Autodesk Inventor part; units mm, degrees
ref_plane "YZ Plane" through (0, 0, 0) normal (1, 0, 0) x (0, 1, 0)
ref_plane "XZ Plane" through (0, 0, 0) normal (0, 1, 0) x (-1, 0, 0)
ref_plane "XY Plane" through (0, 0, 0) normal (0, 0, 1) x (1, 0, 0)
sketch "Sketch1" plane through (0, 0, 0) normal (0, 1, 0) x (-1, 0, 0)
  line L0 (0, 0) -> (50.8, 0)
  line L1 (50.8, 0) -> (50.8, -50.8)
  line L2 (50.8, -50.8) -> (0, -50.8)
  line L3 (0, -50.8) -> (0, 0)
  dimension "d0" = 50.8
  dimension "d1" = 50.8
extrude "Extrusion1" add sketch "Sketch1" along normal blind 3.175
sketch "Sketch2" plane through (0, 3.175, 0) normal (0, 1, 0) x (1, 0, 0)
  line L0 (-50.8, 0) -> (0, 0)
  line L1 (0, 0) -> (0, 50.8)
  line L2 (-50.8, 0) -> (0, 0)
  line L3 (0, 0) -> (0, 3.175)
  line L4 (0, 3.175) -> (-50.8, 3.175)
  line L5 (-50.8, 3.175) -> (-50.8, 0)
  dimension "d4" = 3.175
extrude "Extrusion2" add sketch "Sketch2" along normal blind 22.225
sketch "Sketch3" plane through (0, 3.175, 0) normal (0, 1, 0) x (1, 0, 0)
  line L0 (0, 3.175) -> (0, 50.8)
  line L1 (-50.8, 50.8) -> (-50.8, 3.175)
  line L2 (0, 50.8) -> (-50.8, 50.8)
  point P0 (0, 0)
  point P1 (-12.7, 41.656)
  point P2 (-38.1, 41.656)
  dimension "d9" = 9.144
  dimension "d10" = 9.144
  dimension "d18" = 25.4
  dimension "d19" = 12.7
  dimension "d20" = 12.7
  dimension "d21" = 50.8
hole "Hole1" at (-12.7, 3.175, -41.656) at (-38.1, 3.175, -41.656) direction (0, -1, 0) diameter 6.35 depth 25.4 tip angle 118
sketch "Sketch5" plane through (-50.8, 0, 0) normal (0, 0, 1) x (1, 0, 0)
  line L0 (0, 25.4) -> (50.8, 25.4)
  line L1 (50.8, 0) -> (50.8, 25.4)
  point P0 (25.4, 12.7)
  dimension "d23" = 12.7
  dimension "d24" = 25.4
hole "Hole2" at (-25.4, 12.7, 0) direction (0, 0, -1) diameter 6.35 end through all
properties part number "improved transmission bracket"
Model file for the job. Use its own axes, mm. A direction names the side the tool comes from. Round coordinates to 2 decimals unless told otherwise and drop trailing zeros. Loops run counter-clockwise (first coordinate to the right, second up) from the corner with the lowest first, then second, coordinate; pieces in that order, holes last.
1. Tool access for faces 5 (the cylindrical face through (-39.054, 1.565, -38.628)), 6 (the flat face through (-25, 3.175, -27)): list every direction of +Z, -Z, +X, -X, +Y, -Y with a clear straight run to the whole face (end or side of a thin tool).
Check values:
face 5: +Y, -Y
face 6: -Z, +X, -X, +Y
2. Band-saw the part on A-A, the plane y = 12.7. List the corners of the cut face in (x, z) (3 decimals), and give its area (3 significant figures).
Check values:
outline: (-50.8, -3.175) - (-28.575, -3.175) - (-28.575, 0) - (-50.8, 0) - close; (-22.225, -3.175) - (0, -3.175) - (0, 0) - (-22.225, 0) - close
area: 141 mm2
3. Mould opens along X. For faces 1 (the flat face through (-31, 13, 0)), 2 (the cylindrical face through (-11.484, 1.565, -38.723)), 3 (the flat face through (-50.8, 2, -14)), 4 (the cylindrical face through (-28.55, 13.11, -1.61)) say: +X half, -X half, draft (parallel to the pull), parting line (faces both ways), or undercut.
Check values:
face 1: draft
face 2: undercut
face 3: -X half
face 4: undercut
4. Band-saw the part on B-B, the plane x = -25.4. List the corners of the cut face in (y, z) (3 decimals).
Check values:
outline: (0, -50.8) - (3.175, -50.8) - (3.175, -3.175) - (9.525, -3.175) - (9.525, 0) - (0, 0) - close; (15.875, -3.175) - (25.4, -3.175) - (25.4, 0) - (15.875, 0) - close
5. Wall check: probe 1 along Z at (x, y) = (-38.1, 0.75); probe 2 along Y at (x, z) = (-25.4, -1.05) (3 decimals); probe 3 along Z at (x, y) = (-35, 3.75) (3 decimals). Give the ranges that are in metal, low to high.
Check values:
probe 1: z = -50.8 to -44.83, -38.48 to 0
probe 2: y = 0 to 9.525, 15.875 to 25.4
probe 3: z = -3.175 to 0
6. Band-saw the part on D-D, the plane z = -15.5. List the corners of the cut face in (x, y) (3 decimals), and give its area (3 significant figures).
Check values:
outline: (-50.8, 0) - (0, 0) - (0, 3.175) - (-50.8, 3.175) - close
area: 161 mm2
7. Band-saw the part on C-C, the plane x = -45. List the corners of the cut face in (y, z) (3 decimals), and give its area (3 significant figures).
Check values:
outline: (0, -50.8) - (3.175, -50.8) - (3.175, -3.175) - (25.4, -3.175) - (25.4, 0) - (0, 0) - close
area: 232 mm2
8. Drop flat-ended pins along their axis: P1, Ø14.5, axis at x = -36, z = -29, coming from the +Y side (3 decimals); P2, Ø10, axis at x = -26, y = 20, coming from the -Z side (3 decimals). Give the stop position or say it passes through.
Check values:
P1: stops at y = 3.175
P2: stops at z = -3.175
